```python
from build123d import *

# Parameters (mm, degrees)
CUT_EXTRUDE1_OUTLINE_W                  = 29.05
CUT_EXTRUDE1_OUTLINE_H                  = 42
CUT_EXTRUDE1_DEPTH                      = 10
CUT_EXTRUDE1_START                      = 10
CUT_EXTRUDE1_2_DEPTH                    = 5
CUT_EXTRUDE1_START_2                    = 12.5
CUT_EXTRUDE1_3_DEPTH                    = 2.5
CUT_EXTRUDE1_4_DEPTH                    = 5
CUT_EXTRUDE1_START_3                    = 37
CUT_EXTRUDE1_5_DEPTH                    = 5
BOSS_EXTRUDE1_DEPTH                     = 5
SKETCH3_W                               = 4.5
SKETCH3_H                               = 8.5
CUT_EXTRUDE2_DEPTH                      = 84.790467835
CBORE_FOR_M5_HEX_HEAD_BOLT1_D           = 5.5
CBORE_FOR_M5_HEX_HEAD_BOLT1_CBORE_D     = 13
CBORE_FOR_M5_HEX_HEAD_BOLT1_CBORE_DEPTH = 2
CBORE_FOR_M6_5_SHSS1_D                  = 7.5
CBORE_FOR_M6_5_SHSS1_CBORE_D            = 13
CBORE_FOR_M6_5_SHSS1_CBORE_DEPTH        = 2
SKETCH8_W                               = 2.75
SKETCH8_H                               = 7.5
F_5_5_5_5_DIAMETER_HOLE2_D              = 5.5
F_5_5_5_5_DIAMETER_HOLE2_DEPTH          = 15
CHAMFER2_SIZE                           = 1
CHAMFER3_SIZE                           = 1
CHAMFER4_SIZE                           = 1


with BuildPart() as part:
    # Cut-Extrude1: read off the stored shape, not the designer's step
    # Cut-Extrude1 outline → Cut-Extrude1 (new body)
    with BuildSketch(Plane.YZ):
        with Locations((14.525, 21)):
            Rectangle(CUT_EXTRUDE1_OUTLINE_W, CUT_EXTRUDE1_OUTLINE_H)
    extrude(amount=CUT_EXTRUDE1_DEPTH)

    # Cut-Extrude1 2 outline → Cut-Extrude1 2 (add)
    with BuildSketch(Plane.YZ.offset(CUT_EXTRUDE1_START)):
        Polygon((29.05, 2), (14.05, 2), (14.05, 40), (29.05, 40), (29.05, 42), (0, 42), (0, 0), (29.05, 0), align=None)
    extrude(amount=CUT_EXTRUDE1_2_DEPTH)

    # Cut-Extrude1 3 outline → Cut-Extrude1 3 (add)
    with BuildSketch(Plane.YZ.offset(CUT_EXTRUDE1_START_2)):
        Polygon((14.05, 2), (29.05, 2), (18.080344885, 21), (29.05, 40), (14.05, 40), align=None)
    extrude(amount=CUT_EXTRUDE1_3_DEPTH)

    # Cut-Extrude1 4 outline → Cut-Extrude1 4 (add)
    with BuildSketch(Plane.XY):
        Polygon((0, 29.05), (-15, 0), (0, 0), align=None)
    extrude(amount=CUT_EXTRUDE1_4_DEPTH)

    # Cut-Extrude1 5 outline → Cut-Extrude1 5 (add)
    with BuildSketch(Plane.XY.offset(CUT_EXTRUDE1_START_3)):
        Polygon((0, 29.05), (-15, 0), (0, 0), align=None)
    extrude(amount=CUT_EXTRUDE1_5_DEPTH)

    # Sketch2 → Boss-Extrude1 (add)
    with BuildSketch(Plane.XZ):
        with BuildLine():
            Line((-9.113819566, -14.079577983), (-44.613819566, 46.120422017))
            ThreePointArc((-44.613819566, 46.120422017), (-43.61404549, 57.68277034), (-32.359107934, 60.513640801))
            Line((-32.359107934, 60.513640801), (15, 42))
            Line((15, 42), (15, 0))
            Line((15, 0), (8.492070756, -13.375232968))
            ThreePointArc((8.492070756, -13.375232968), (-0.100257626, -18.992007107), (-9.113819566, -14.079577983))
        make_face()
    extrude(amount=BOSS_EXTRUDE1_DEPTH)

    # Sketch3 → Cut-Extrude2 (cut, through all)
    with BuildSketch(Plane.XZ.offset(5)):
        with Locations((5.25, 21)):
            Rectangle(SKETCH3_W, SKETCH3_H)
    extrude(amount=-CUT_EXTRUDE2_DEPTH, mode=Mode.SUBTRACT)

    # CBORE for M5 Hex Head Bolt1 (through all)
    with Locations(Plane(origin=(0, 0, 0), x_dir=(1, 0, 0), z_dir=(0, 1, 0))):
        with Locations((-0.5, 9)):
            CounterBoreHole(CBORE_FOR_M5_HEX_HEAD_BOLT1_D / 2, CBORE_FOR_M5_HEX_HEAD_BOLT1_CBORE_D / 2, CBORE_FOR_M5_HEX_HEAD_BOLT1_CBORE_DEPTH)

    # CBORE for M6.5 SHSS1 (through all)
    with Locations(Plane(origin=(0, 0, 0), x_dir=(1, 0, 0), z_dir=(0, 1, 0))):
        with Locations((-36, -51.2)):
            CounterBoreHole(CBORE_FOR_M6_5_SHSS1_D / 2, CBORE_FOR_M6_5_SHSS1_CBORE_D / 2, CBORE_FOR_M6_5_SHSS1_CBORE_DEPTH)

    # Sketch8 → Ø5.5 (5.5) Diameter Hole1 (revolve, cut)
    with BuildSketch(Plane(origin=(7.5, 10.55, 21), x_dir=(0, 0, 1), z_dir=(0, 1, 0))):
        with Locations((1.375, 3.75)):
            Rectangle(SKETCH8_W, SKETCH8_H)
    revolve(axis=Axis((1.15, 10.55, 21), (1, 0, 0)), mode=Mode.SUBTRACT)

    # Ø5.5 (5.5) Diameter Hole2
    with Locations(Plane.ZY):
        with Locations((21, 10.55)):
            Hole(F_5_5_5_5_DIAMETER_HOLE2_D / 2, depth=F_5_5_5_5_DIAMETER_HOLE2_DEPTH)

    # Chamfer2
    chamfer2_edges = [part.edges().sort_by_distance(p)[0] for p in [
        (-7.5, 14.525, 42),
        (7.5, 29.05, 42),
        (-7.5, 14.525, 5),
        (7.5, 29.05, 0),
        (-7.5, 14.525, 0),
        (-7.5, 14.525, 37),
        (-0.100257626, 0, -18.992007107),
        (11.746035378, 0, -6.687616484),
        (-8.679553967, 0, 51.2568204),
        (-43.61404549, 0, 57.68277034),
        (-26.863819566, 0, 16.020422017),
    ]]
    chamfer(chamfer2_edges, length=CHAMFER2_SIZE)

    # Chamfer3
    chamfer3_edges = [part.edges().sort_by_distance(p)[0] for p in [
        (0, 29.05, 21),
    ]]
    chamfer(chamfer3_edges, length=CHAMFER3_SIZE)

    # Chamfer4
    chamfer4_edges = [part.edges().sort_by_distance(p)[0] for p in [
        (15, 13.525, 0),
        (15, 13.525, 42),
    ]]
    chamfer(chamfer4_edges, length=CHAMFER4_SIZE)


solid = part.part
```
Work out the finished part from the listing and answer in its coordinate system (mm). A direction names the side the tool comes from. Give positions to 0.01 mm unless a question says otherwise; leave off trailing zeros. Write each loop counter-clockwise with the first axis right and the second up, starting at its lowest first coordinate (ties: lowest second). Pieces come first, ordered by that corner, then holes. Notation, with made-up numbers: (36.5, -24.75) -> (44.5, -24.75) arc R21 cw to (44.5, 3.25) -> close; hole circle Ø1 at (8.5, -35.75). An arc over 180 degrees is marked (long way). Write each question's results on one line, items separated by ' | '.
1. Find section A-A on x = -36. Determine the outline of the cut face in (y, z).
Data:
outline: (-5, 31.51) -> (-1, 31.51) -> (0, 33.48) -> (0, 44.7) -> (-2, 44.7) -> (-2, 47.45) -> (-5, 47.45) -> close; (-5, 54.95) -> (-2, 54.95) -> (-2, 57.7) -> (0, 57.7) -> (0, 60.2) -> (-1, 61.2) -> (-5, 61.2) -> close
2. Each of these flat-tipped pins is pushed along its axis until it touches: pin 1 Ø6 at (x, y) = (2, 21) entering from +Z; pin 2 Ø4 at (x, y) = (-6, 9) entering from -Z; pin 3 Ø9.5 at (y, z) = (19, 20.5) entering from -X; pin 4 Ø5 at (y, z) = (10.55, 21) entering from -X. Where does it stop, or does it pass through?
Data:
pin 1: z = 42 | pin 2: z = 0 | pin 3: x = 0 | pin 4: through
3. Determine the mould class of faces 1 (the conical face through (-43.087, -0.174, 57.025)), 2 (the flat face through (3, 12, 24)), 3 (the flat face through (-18, 0, 24)), 4 (the cylindrical face through (-1.346, -0.986, -15.445)) for opening direction X: +X half, -X half, draft (parallel to the pull), parting line (faces both ways), or undercut.
Data:
face 1: parting line | face 2: undercut | face 3: draft | face 4: undercut
4. Find section C-C on z = 51.2. Determine the outline of the cut face in (x, y), and give its area (3 significant figures).
Data:
outline: (-46, -5) -> (-39.75, -5) -> (-39.75, -2) -> (-42.5, -2) -> (-42.5, 0) -> (-45, 0) -> (-46, -1) -> close; (-32.25, -5) -> (-8.53, -5) -> (-8.53, -1) -> (-11.28, 0) -> (-29.5, 0) -> (-29.5, -2) -> (-32.25, -2) -> close | area: 137 mm^2
5. A tool of negligible diameter and unlimited length cuts with its end or side. For faces 5 (the flat face through (-6.85, 14.71, 4.49)), 6 (the flat face through (3, 11, 0)), 7 (the flat face through (10, 21, 21)), from which of +Z, -Z, +X, -X, +Y, -Y can it reach the whole face along a straight path? Write none if from no direction.
Data:
face 5: -X, +Y | face 6: -Z, +X, -X, +Y | face 7: +Y
6. Find section B-B on y = 22. Determine the outline of the cut face in (x, z).
Data:
outline: (-3.64, 1) -> (-2.51, 0) -> (14, 0) -> (15, 1) -> (15, 14.21) -> (12.5, 14.21) -> (12.5, 2) -> (10, 2) -> (10, 40) -> (12.5, 40) -> (12.5, 27.79) -> (15, 27.79) -> (15, 41) -> (14, 42) -> (-2.51, 42) -> (-3.64, 41) -> (-3.64, 38) -> (-2.51, 37) -> (0, 37) -> (0, 5) -> (-2.51, 5) -> (-3.64, 4) -> close; hole (3, 16.75) -> (7.5, 16.75) -> (7.5, 25.25) -> (3, 25.25) -> close
7. Straight lines are drawn through the part: L1, parallel to Y at x = 10.75, z = 21; L2, parallel to Z at x = 6, y = 21; L3, parallel to X at y = 8, z = 17. For each, find the intervals that lie inside material, in ascending order.
Data:
L1: -5 to 7.8, 13.3 to 14.05 | L2: 0 to 16.75, 25.25 to 42 | L3: 0 to 3, 7.5 to 15
8. Find section D-D on y = 10.55. Determine the outline of the cut face in (x, z), and give its area (3 significant figures).
Data:
outline: (-9.55, 1) -> (-8.43, 0) -> (14, 0) -> (15, 1) -> (15, 18.25) -> (7.5, 18.25) -> (7.5, 16.75) -> (3, 16.75) -> (3, 18.25) -> (0, 18.25) -> (0, 5) -> (-8.43, 5) -> (-9.55, 4) -> close; (-9.55, 38) -> (-8.43, 37) -> (0, 37) -> (0, 23.75) -> (3, 23.75) -> (3, 25.25) -> (7.5, 25.25) -> (7.5, 23.75) -> (15, 23.75) -> (15, 41) -> (14, 42) -> (-8.43, 42) -> (-9.55, 41) -> close | area: 626 mm^2
